Here's how the part is built. I have some questions about the finished solid (model axes, mm). Face numbers are marked on the shaded views. A direction names the side the tool comes from. Round coordinates to 2 decimals unless told otherwise and drop trailing zeros. Order: outer loops, then holes, each group sorted by start corner. A loop starts at its lowest first (then second) coordinate and runs counter-clockwise, first axis right, second up. Notation, with made-up numbers: (37.25, 19.25) -> (55.25, 19.25) arc R27 cw to (55.25, 39.25) -> close; hole circle Ø1 at (-16.75, -39.75). An arc over 180 degrees is marked (long way). Use a Markdown table: item, result. Add a question column.
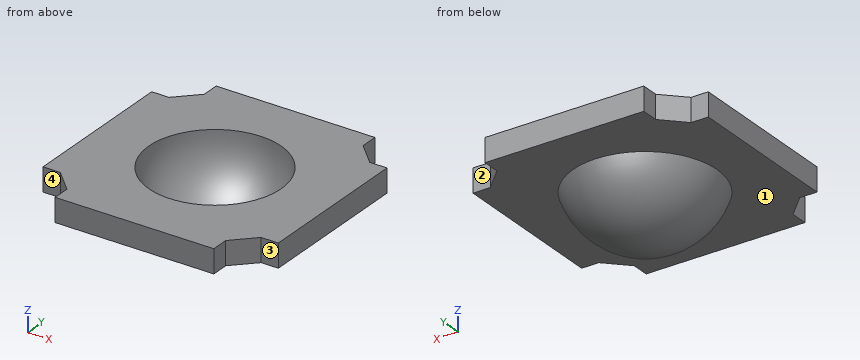
Autodesk Inventor part; units mm, degrees
ref_plane "YZ Plane" through (0, 0, 0) normal (1, 0, 0) x (0, 1, 0)
ref_plane "XZ Plane" through (0, 0, 0) normal (0, 1, 0) x (-1, 0, 0)
ref_plane "XY Plane" through (0, 0, 0) normal (0, 0, 1) x (1, 0, 0)
sketch "Sketch1" plane through (0, 0, 0) normal (0, 0, 1) x (1, 0, 0)
  line L0 (-38.8739, 0) -> (58.9391, 0) construction
  line L1 (0, -36.2399) -> (0, 43.1348) construction
  line L2 (0, 0) -> (31.7956, 31.7956) construction
  line L3 (0, 0) -> (44.9658, 0) construction
  line L4 (0, 24.9006) -> (16.8, 24.9006)
  line L5 (16.8, 24.9006) -> (16.8, 21.2406)
  line L6 (16.8, 21.2406) -> (19.0203, 19.0203)
  line L7 (24.9006, 0) -> (24.9006, 16.8)
  line L8 (24.9006, 16.8) -> (21.2406, 16.8)
  line L9 (21.2406, 16.8) -> (19.0203, 19.0203)
  line L10 (0, 24.9006) -> (-16.8, 24.9006)
  line L11 (-16.8, 24.9006) -> (-16.8, 21.2406)
  line L12 (-16.8, 21.2406) -> (-19.0203, 19.0203)
  line L13 (-24.9006, 0) -> (-24.9006, 16.8)
  line L14 (-24.9006, 16.8) -> (-21.2406, 16.8)
  line L15 (-21.2406, 16.8) -> (-19.0203, 19.0203)
  line L16 (0, -24.9006) -> (16.8, -24.9006)
  line L17 (16.8, -24.9006) -> (16.8, -21.2406)
  line L18 (16.8, -21.2406) -> (19.0203, -19.0203)
  line L19 (24.9006, 0) -> (24.9006, -16.8)
  line L20 (24.9006, -16.8) -> (21.2406, -16.8)
  line L21 (21.2406, -16.8) -> (19.0203, -19.0203)
  line L22 (0, -24.9006) -> (-16.8, -24.9006)
  line L23 (-16.8, -24.9006) -> (-16.8, -21.2406)
  line L24 (-16.8, -21.2406) -> (-19.0203, -19.0203)
  line L25 (-24.9006, 0) -> (-24.9006, -16.8)
  line L26 (-24.9006, -16.8) -> (-21.2406, -16.8)
  line L27 (-21.2406, -16.8) -> (-19.0203, -19.0203)
  circle A0 centre (0, 0) radius 14
  dimension "d0" = 45
  dimension "d1" = 16.8
  dimension "d2" = 3.66
  dimension "d3" = 3.14
  dimension "d4" = 28
extrude "Extrusion1" add sketch "Sketch1" along normal blind 5
sketch "Sketch2" plane through (0, 0, 5) normal (0, 0, 1) x (1, 0, 0)
  circle A0 centre (0, 0) radius 14 construction
  line L0 (16.8, 24.9006) -> (-16.8, 24.9006) construction
  line L1 (-16.8, 24.9006) -> (-16.8, 21.2406) construction
  line L2 (-16.8, 21.2406) -> (-21.2406, 16.8) construction
  line L3 (-21.2406, 16.8) -> (-24.9006, 16.8) construction
  line L4 (-24.9006, 16.8) -> (-24.9006, -16.8) construction
  line L5 (-24.9006, -16.8) -> (-21.2406, -16.8) construction
  line L6 (-21.2406, -16.8) -> (-16.8, -21.2406) construction
  line L7 (-16.8, -21.2406) -> (-16.8, -24.9006) construction
  line L8 (-16.8, -24.9006) -> (16.8, -24.9006) construction
  line L9 (16.8, -24.9006) -> (16.8, -21.2406) construction
  line L10 (16.8, -21.2406) -> (21.2406, -16.8) construction
  line L11 (21.2406, -16.8) -> (24.9006, -16.8) construction
  line L12 (24.9006, -16.8) -> (24.9006, 16.8) construction
  line L13 (24.9006, 16.8) -> (21.2406, 16.8) construction
  line L14 (21.2406, 16.8) -> (16.8, 21.2406) construction
  line L15 (16.8, 21.2406) -> (16.8, 24.9006) construction
  line L16 (-34.8609, 0) -> (34.8609, 0) construction
  line L17 (0, -34.8609) -> (0, 34.8609) construction
  circle A1 centre (13, -13) radius 2.5
  circle A2 centre (-13, -13) radius 2.5
  dimension "d7" = 5
  dimension "d8" = 13
  dimension "d9" = 13
extrude "Extrusion2" [suppressed]
sketch "Sketch3" plane through (0, 0, 0) normal (1, 0, 0) x (0, 1, 0)
  line L0 (-14, 5) -> (14, 5) construction
  line L1 (24.9006, 5) -> (21.2406, 5) construction
  line L2 (21.2406, 5) -> (16.8, 5) construction
  line L3 (16.8, 5) -> (-16.8, 5) construction
  line L4 (-16.8, 5) -> (-21.2406, 5) construction
  line L5 (-21.2406, 5) -> (-24.9006, 5) construction
  line L6 (-24.9006, 5) -> (-21.2406, 5) construction
  line L7 (-21.2406, 5) -> (-16.8, 5) construction
  line L8 (-16.8, 5) -> (16.8, 5) construction
  line L9 (16.8, 5) -> (21.2406, 5) construction
  line L10 (21.2406, 5) -> (24.9006, 5) construction
  line L11 (24.9006, 0) -> (21.2406, 0) construction
  line L12 (24.9006, 0) -> (24.9006, 5) construction
  line L13 (21.2406, 5) -> (24.9006, 5) construction
  line L14 (21.2406, 0) -> (21.2406, 5) construction
  line L15 (21.2406, 0) -> (16.8, 0) construction
  line L16 (21.2406, 0) -> (21.2406, 5) construction
  line L17 (16.8, 5) -> (21.2406, 5) construction
  line L18 (16.8, 0) -> (16.8, 5) construction
  line L19 (16.8, 0) -> (-16.8, 0) construction
  line L20 (16.8, 0) -> (16.8, 5) construction
  line L21 (-16.8, 5) -> (16.8, 5) construction
  line L22 (-16.8, 0) -> (-16.8, 5) construction
  line L23 (-16.8, 0) -> (-21.2406, 0) construction
  line L24 (-16.8, 0) -> (-16.8, 5) construction
  line L25 (-21.2406, 5) -> (-16.8, 5) construction
  line L26 (-21.2406, 0) -> (-21.2406, 5) construction
  line L27 (-21.2406, 0) -> (-24.9006, 0) construction
  line L28 (-21.2406, 0) -> (-21.2406, 5) construction
  line L29 (-24.9006, 5) -> (-21.2406, 5) construction
  line L30 (-24.9006, 0) -> (-24.9006, 5) construction
  line L31 (-14, 5) -> (14, 5) construction
  line L32 (14, 0) -> (-14, 0) construction
  line L33 (16.8, 5) -> (-16.8, 5)
  arc A0 (0, -9) -> (14, 5) centre (0, 5) ccw
  line L34 (0, -16.0037) -> (0, 8.5006) construction
  arc A1 (0, -11) -> (16, 5) centre (0, 5) ccw
  line L35 (0, -9) -> (0, -11)
  line L36 (16, 5) -> (14, 5)
revolve "Revolution1" add sketch "Sketch3" angle 360 about axis through (0, 0, -10) along (0, 0, 1)
equation "\"d9\" = d8"
properties part number "20_Cube_Insert_Eye"
(1) I want a section at A-A on z = 3.5. List the corners of the cut face in (x, y) for me.
(2) I'm going to push flat-ended pins straight in: P1, Ø1.1, axis at y = 23, z = 2, coming from the +X side; P2, Ø3, axis at x = 14, y = -19.5, coming from the -Z side; P3, Ø3, axis at x = 23, z = 2.5, coming from the +Y side. Where does each tip first touch, or does it pass through?
(3) I want a section at D-D on y = -16. List the corners of the cut face in (x, z) for me, and give its area (3 significant figures).
(4) I want a section at C-C on x = 5. List the corners of the cut face in (y, z) for me.
(5) Please list where these lines run through material, in increasing order: probe 1 along Y at (x, z) = (2, -6); probe 2 along Y at (x, z) = (6.5, -0.5); probe 3 along Y at (x, z) = (22.5, 3.25). Write a range as from..to.
(6) I want a section at B-B on y = 3. List the corners of the cut face in (x, z) for me, and give its area (3 significant figures).
(7) On a 3-axis mill with a long thin cutter (end or side, diameter ignored), from which of +Z, -Z, +X, -X, +Y, -Y can I reach the whole of each face in a straight line? I mean the marked faces 1, 2, 3 and 4. Say none if no direction works.
Output:
| question | item | result |
|---|---|---|
| 1 | outline | (-24.9, -16.8) -> (-21.24, -16.8) -> (-16.8, -21.24) -> (-16.8, -24.9) -> (16.8, -24.9) -> (16.8, -21.24) -> (21.24, -16.8) -> (24.9, -16.8) -> (24.9, 16.8) -> (21.24, 16.8) -> (16.8, 21.24) -> (16.8, 24.9) -> (-16.8, 24.9) -> (-16.8, 21.24) -> (-21.24, 16.8) -> (-24.9, 16.8) -> close; hole circle Ø27.84 at (0, 0) |
| 2 | P1 | x = 16.8 |
| 2 | P2 | z = 0 |
| 2 | P3 | y = 16.8 |
| 3 | outline | (-24.9, 0) -> (24.9, 0) -> (24.9, 5) -> (-24.9, 5) -> close |
| 3 | area | 249 mm² |
| 4 | outline | (-24.9, 0) -> (-14.35, 0) arc R15.2 ccw to (14.35, 0) -> (24.9, 0) -> (24.9, 5) -> (13.08, 5) arc R13.08 cw to (-13.08, 5) -> (-24.9, 5) -> close |
| 5 | probe 1 | -11.45..-8.43, 8.43..11.45 |
| 5 | probe 2 | -13.55..-11.11, 11.11..13.55 |
| 5 | probe 3 | -16.8..16.8 |
| 6 | outline | (-24.9, 0) -> (-14.9, 0) arc R15.72 ccw to (14.9, 0) -> (24.9, 0) -> (24.9, 5) -> (13.67, 5) arc R13.67 cw to (-13.67, 5) -> (-24.9, 5) -> close |
| 6 | area | 189 mm² |
| 7 | face 1 | -Z |
| 7 | face 2 | +Z, -Z, +X, +Y |
| 7 | face 3 | +Z, -Z, +X, -Y |
| 7 | face 4 | +Z, -Z, -X, -Y |
